Check sheet for the modelled part. Datum: model origin and axes. Units: mm. Coordinates: 2 decimals unless noted, no trailing zeros. Loops run counter-clockwise (first coordinate to the right, second up) from the corner with the lowest first, then second, coordinate; pieces in that order, holes last. Notation, with made-up numbers: (81, -13.75) -> (92, -13.75) arc R14 ccw to (92, 9.25) -> close; hole circle Ø2 at (70, 82). An arc over 180 degrees is marked (long way). Use CSV: the item, a comma, the result in double quotes.
Autodesk Inventor part; units mm, degrees
ref_plane "Work Plane2" through (178, -56.0619, -70.2985) normal (1, 0, 0) x (0, 0.8411785, -0.5407576)
ref_plane "YZ Plane" through (0, 0, 0) normal (1, 0, 0) x (0, 1, 0)
ref_plane "XZ Plane" through (0, 0, 0) normal (0, 1, 0) x (-1, 0, 0)
ref_plane "Work Plane1" through (0, 4.7283, -22.9522) normal (-1, 0, 0) x (0, -0.8411785, 0.5407576)
sketch "Sketch1" plane through (0, 4.7283, -22.9522) normal (-1, 0, 0) x (0, -0.8411785, 0.5407576)
  line L0 (61.5, -12.25) -> (61.5, -16.75)
  line L1 (61.5, -16.75) -> (65.5, -16.75)
  line L2 (65.5, -16.75) -> (65.5, -20.25)
  line L3 (65.5, -20.25) -> (79.5, -20.25)
  line L4 (79.5, -20.25) -> (65.5, -11.25)
  line L5 (65.5, -11.25) -> (65.5, -12.25)
  line L6 (65.5, -12.25) -> (61.5, -12.25)
  line L7 (16.3889, 16.75) -> (16.3889, 18.75)
  line L8 (14.7421, 12.75) -> (16.3889, 18.75)
  line L9 (64.2739, -12.25) -> (12.3502, 21.1295)
  line L10 (16.3889, 16.75) -> (16.3889, 18.5332)
  arc A0 (-57.551, -16.75) -> (-61.5, -12.801) centre (-58.75, -14) ccw
  arc A1 (-34.301, -16.75) -> (-36.699, -16.75) centre (-35.5, -14) ccw
  line L11 (61.5, -12.25) -> (16.3889, 16.75)
  line L12 (16.3889, 13.75) -> (-61.5, 13.75)
  line L13 (-61.5, 13.75) -> (-61.5, -12.801)
  line L14 (-61.5, 13.75) -> (-61.5, -12.801)
  arc A2 (-57.551, -16.75) -> (-61.5, -12.801) centre (-58.75, -14) ccw
  line L15 (-57.551, -16.75) -> (-36.699, -16.75)
  arc A3 (-34.301, -16.75) -> (-36.699, -16.75) centre (-35.5, -14) ccw
  line L16 (-34.301, -16.75) -> (61.5, -16.75)
  line L17 (61.5, -16.75) -> (61.5, -12.25)
  line L18 (21.0556, 13.75) -> (-61.5, 13.75)
  line L19 (-57.551, -16.75) -> (-36.699, -16.75)
  line L20 (-34.301, -16.75) -> (61.5, -16.75)
  line L21 (61.5, -16.75) -> (61.5, -12.25)
  line L22 (61.5, -12.25) -> (21.0556, 13.75)
  point P0 (16.3889, 18.5332)
  point P1 (15.5655, 15.75)
  point P2 (16.3889, 18.5332)
  point P3 (16.3383, 18.5657)
  dimension "d14" = 1.5
  dimension "d15" = 2
ref_plane "Work Plane2" through (178, -56.0619, -70.2985) normal (1, 0, 0) x (0, 0.8411785, -0.5407576)
extrude "Extrusion1" add sketch "Sketch1" against normal up to surface (178 mm away) contours L11 L7 L9 L6
sketch "Sketch2" plane through (0, -55.9618, 1.5) normal (0, 0, 1) x (1, 0, 0)
  circle A0 centre (3, 16.4427) radius 2.5
  circle A1 centre (3, 35.7569) radius 2.5
  line L0 (0, 2.3333) -> (0, 55.9618)
  line L1 (0, 2.3333) -> (3, 2.3333)
  line L2 (6, 50.414) -> (6, 9.4662)
  line L3 (0, 50.414) -> (6, 50.414)
  circle A2 centre (175, 21.9904) radius 2.5
  circle A3 centre (175, 41.3047) radius 2.5
  line L4 (178, 2.3333) -> (178, 55.9618)
  line L5 (178, 55.9618) -> (172, 55.9618)
  line L6 (172, 55.9618) -> (172, 2.3333)
  line L7 (178, 2.3333) -> (172, 2.3333)
  line L8 (3, 9.4662) -> (3, 2.3333)
  line L9 (3, 9.4662) -> (6, 9.4662)
  point P0 (3, 35.7569)
  point P1 (3, 16.4427)
hole "Hole1" at (3, -20.2049, 1.5) at (3, -39.5191, 1.5) at (175, -33.9713, 1.5) at (175, -14.6571, 1.5) direction (0, 0, -1) diameter 3.6 end through all countersink diameter 7 countersink angle 90
ref_plane "Work Plane3" through (22, -31.0502, -8.6656) normal (0, -0.7712334, 0.6365525) x (1, 0, 0)
sketch "Sketch3" plane through (22, -31.0502, -8.6656) normal (0, -0.7712334, 0.6365525) x (1, 0, 0)
  line L0 (-9.9215, 5.3729) -> (-9.9215, -5.5323)
  spline S0 degree 3 poles (-9.9215, -5.5323) (-9.9222, -5.6561) (-9.8204, -5.8999) (-9.5772, -6.0011) (-9.4534, -6.0004) knots 0 0 0 0 0.5 1 1 1 1
  line L1 (-9.4534, -6.0004) -> (19.4534, -6.0004)
  spline S1 degree 3 poles (19.4534, -6.0004) (19.5775, -6.0011) (19.8219, -5.8989) (19.9222, -5.6548) (19.9215, -5.5307) knots 0 0 0 0 0.5 1 1 1 1
  line L2 (19.9215, -5.5307) -> (19.9215, 5.3744)
  spline S2 degree 3 poles (19.9215, 5.3744) (19.9222, 5.4985) (19.82, 5.743) (19.5758, 5.8433) (19.4518, 5.8426) knots 0 0 0 0 0.5 1 1 1 1
  line L3 (19.4518, 5.8426) -> (-9.4534, 5.8426)
  spline S3 degree 3 poles (-9.4534, 5.8426) (-9.5775, 5.8433) (-9.8219, 5.7411) (-9.9222, 5.4969) (-9.9215, 5.3729) knots 0 0 0 0 0.5 1 1 1 1
  circle A0 centre (-8.3791, -4.458) radius 0.5
  circle A1 centre (-8.3791, 4.3001) radius 0.5
  circle A2 centre (18.3791, 4.3001) radius 0.5
  circle A3 centre (18.3791, -4.458) radius 0.5
  arc A4 (5.2617, -1.5301) -> (5.1811, -1.6008) centre (5.2771, -1.6289) ccw
  arc A5 (5.1811, 1.4429) -> (5.1811, -1.6008) centre (0, -0.0789) ccw
  arc A6 (5.1811, 1.4429) -> (5.2617, 1.3723) centre (5.2771, 1.4711) ccw
  arc A7 (5.2617, 1.3723) -> (5.3414, 1.4401) centre (5.2463, 1.4711) ccw
  arc A8 (5.3414, -1.5979) -> (5.3414, 1.4401) centre (10, -0.0789) ccw
  arc A9 (5.3414, -1.5979) -> (5.2617, -1.5301) centre (5.2463, -1.6289) ccw
  line L4 (143.9215, 5.3729) -> (143.9215, -5.5323)
  spline S4 degree 3 poles (143.4534, 5.8426) (143.5775, 5.8433) (143.8219, 5.7411) (143.9222, 5.4969) (143.9215, 5.3729) knots 0 0 0 0 0.5 1 1 1 1
  line L5 (114.5482, 5.8426) -> (143.4534, 5.8426)
  spline S5 degree 3 poles (114.0785, 5.3744) (114.0778, 5.4985) (114.18, 5.743) (114.4242, 5.8433) (114.5482, 5.8426) knots 0 0 0 0 0.5 1 1 1 1
  line L6 (114.0785, -5.5307) -> (114.0785, 5.3744)
  spline S6 degree 3 poles (114.5466, -6.0004) (114.4225, -6.0011) (114.1781, -5.8989) (114.0778, -5.6548) (114.0785, -5.5307) knots 0 0 0 0 0.5 1 1 1 1
  line L7 (143.4534, -6.0004) -> (114.5466, -6.0004)
  spline S7 degree 3 poles (143.9215, -5.5323) (143.9222, -5.6561) (143.8204, -5.8999) (143.5772, -6.0011) (143.4534, -6.0004) knots 0 0 0 0 0.5 1 1 1 1
  circle A10 centre (142.3791, -4.458) radius 0.5
  circle A11 centre (142.3791, 4.3001) radius 0.5
  circle A12 centre (115.6209, 4.3001) radius 0.5
  circle A13 centre (115.6209, -4.458) radius 0.5
  arc A14 (128.8189, -1.6008) -> (128.7383, -1.5301) centre (128.7229, -1.6289) ccw
  arc A15 (128.7383, -1.5301) -> (128.6586, -1.5979) centre (128.7537, -1.6289) ccw
  arc A16 (128.6586, 1.4401) -> (128.6586, -1.5979) centre (124, -0.0789) ccw
  arc A17 (128.6586, 1.4401) -> (128.7383, 1.3723) centre (128.7537, 1.4711) ccw
  arc A18 (128.7383, 1.3723) -> (128.8189, 1.4429) centre (128.7229, 1.4711) ccw
  arc A19 (128.8189, -1.6008) -> (128.8189, 1.4429) centre (134, -0.0789) ccw
  circle A20 centre (10, -0.0789) radius 5.4
  circle A21 centre (124, -0.0789) radius 5.4
  line L8 (0, 5.3211) -> (10, 5.3211)
  line L9 (10, -5.4789) -> (0, -5.4789)
  line L10 (124, 5.3211) -> (134, 5.3211)
  line L11 (134, -5.4789) -> (124, -5.4789)
  point P0 (-22, 26.4483)
  point P1 (14.6373, -1.6617)
  point P2 (5, 1.9607)
  point P3 (5.3627, -1.6617)
  point P4 (5, -2.1185)
  point P5 (7.5029, -4.2949)
  point P6 (3.3743, -4.2949)
  point P7 (5.2923, -1.5401)
  dimension "d9" = 10.8
  dimension "d10" = 10.8
extrude "Extrusion2" cut sketch "Sketch3" along normal blind 78.25 contours A9 A8 A7 A6 A5 A20 A4 | A4 A5 A20 A6 A7 A8 A9 | A5 A20 | A19 A21 A18 A17 A16 A15 A14 | A14 A15 A16 A17 A18 A19 A21 | A21 A19 | A19 L11 A21 | A19 A21 L10
properties part number "front" material "Aluminum 6061"
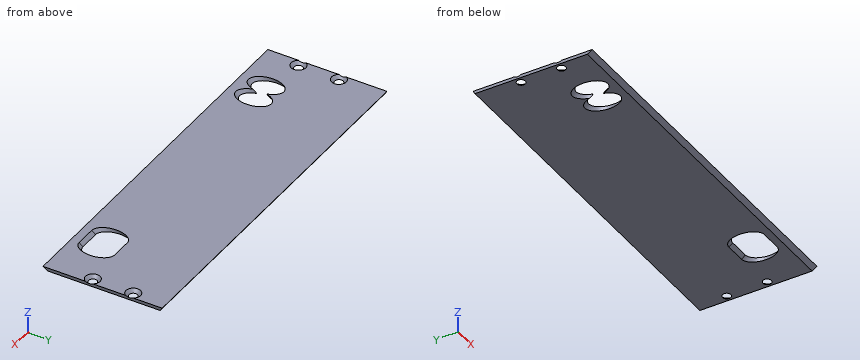
1) Cross-section at D-D on x = 35. Record the boundary of the cut face in (y, z), and give its area (3 significant figures).
Answer below:
outline,"(-55.96, 1.5) -> (-53.63, 0) -> (-48.73, 0) -> (-50.54, 1.5) -> close; (-36.44, 1.5) -> (-34.62, 0) -> (0, 0) -> (0.96, 1.5) -> close"
area,"61.8 mm²"
2) Cross-section at B-B on x = 3. Record the boundary of the cut face in (y, z), and give its area (3 significant figures).
Answer below:
outline,"(-55.96, 1.5) -> (-53.63, 0) -> (-41.52, 0) -> (-43.02, 1.5) -> close; (-37.52, 0) -> (-22.2, 0) -> (-23.7, 1.5) -> (-36.02, 1.5) -> close; (-18.2, 0) -> (0, 0) -> (0.96, 1.5) -> (-16.7, 1.5) -> close"
area,"66.4 mm²"
3) Cross-section at A-A on x = 152.5. Record the boundary of the cut face in (y, z).
Answer below:
outline,"(-55.96, 1.5) -> (-53.63, 0) -> (-50.16, 0) -> (-51.97, 1.5) -> close; (-35.01, 1.5) -> (-33.19, 0) -> (0, 0) -> (0.96, 1.5) -> close"
4) Thickness scan on line 1 along X through (y, z) = (-38.5, 0.9); line 2 along X through (y, z) = (-49.5, 0.3); line 3 along X through (y, z) = (-40.5, 0.9). Record the ranges inside material, lowest first. Write a range as from..to.
Answer below:
line 1,"x = 0..0.28, 5.72..17.33, 26.67..27.33, 36.67..141.33, 160.67..178"
line 2,"x = 0..19.43, 24.57..29.43, 34.57..143.43, 158.57..178"
line 3,"x = 0..0.27, 5.73..16.8, 37.2..140.8, 161.2..178"
5) Cross-section at C-C on z = 0.5. Give the number of separate pieces and of enclosed holes in the cut face, and give its area (3 significant figures).
Answer below:
separate pieces,"1"
enclosed holes,"6"
area,"9,070 mm²"
